```python
from build123d import *

# Parameters (mm, degrees)
EXTRUDE_1_DEPTH     = 5
SKETCH_2_W          = 5.436001784
SKETCH_2_H          = 4
CUT_EXTRUDE_1_DEPTH = 0.3
FILLET_2_R          = 0.3
EXTRUDE_2_DEPTH     = 5


with BuildPart() as part:
    # 草图1 → 凸台-拉伸1 (new body)
    with BuildSketch(Plane.XY):
        with BuildLine():
            Line((-6.127180226, -2.201181898), (-3.631722259, 2.12107809))
            ThreePointArc((-3.631722259, 2.12107809), (-3.262353303, 2.018731118), (-3.073540248, 1.685177587))
            Line((-3.073540248, 1.685177587), (1.998975947, -2.27609726))
            Line((1.998975947, -2.27609726), (6.288373272, -9.705551361))
            Line((6.288373272, -9.705551361), (7.418073814, -11.662250097))
            Line((7.418073814, -11.662250097), (2.221921391, -14.662250097))
            Line((2.221921391, -14.662250097), (-4.395129419, -3.201181898))
            Line((-4.395129419, -3.201181898), (-6.127180226, -2.201181898))
        make_face()
    extrude(amount=EXTRUDE_1_DEPTH)

    # 草图2 → 切除-拉伸1 (cut)
    with BuildSketch(Plane(origin=(-0.346861308, -0.444164989, 0), x_dir=(0.7881471083112889, -0.6154869094144516, 0), z_dir=(0.6154869094144517, 0.788147108311289, 0))):
        with Locations((-0.241605711, -2.5)):
            Rectangle(SKETCH_2_W, SKETCH_2_H)
    extrude(amount=-CUT_EXTRUDE_1_DEPTH, mode=Mode.SUBTRACT)

    # 圆角2
    fillet_2_edges = [part.edges().sort_by_distance(p)[0] for p in [
        (-2.864112767, 1.14099, 2.5),
        (-0.721928223, -0.531903969, 0.5),
        (1.42025632, -2.204797938, 2.5),
        (-0.721928223, -0.531903969, 4.5),
    ]]
    fillet(fillet_2_edges, radius=FILLET_2_R - 0.0001)  # a hair under: the kernel refuses the full size

    # 草图3 → 凸台-拉伸2 (add)
    with BuildSketch(Plane.XY.offset(5)):
        Polygon((7.418073814, -11.662250097), (15.362099483, -16.248735455), (13.872535789, -18.828735455), (4.438946425, -13.382250097), align=None)
    extrude(amount=-EXTRUDE_2_DEPTH)


solid = part.part
```
Build history of the part. All positions in model axes, mm. A direction names the side the tool comes from. Give positions to 0.01 mm unless a question says otherwise; leave off trailing zeros. Loops run counter-clockwise (first coordinate to the right, second up) from the corner with the lowest first, then second, coordinate; pieces in that order, holes last. Notation, with made-up numbers: (27.5, -39.75) -> (44.5, -39.75) arc R27 cw to (44.5, -12.75) -> close; hole circle Ø1 at (25.25, 76.5). An arc over 180 degrees is marked (long way). One line per question, with ' | ' between items.
Q1. Tool access for faces 1 (the flat face through (3.35, -14.01, 2.46)), 2 (the flat face through (-4.897, -0.07, 2.465)): list every direction of +Z, -Z, +X, -X, +Y, -Y with a clear straight run to the whole face (end or side of a thin tool).
Filled sheet:
face 1: +Z, -Z, -Y | face 2: +Z, -Z, -X, +Y
Q2. Drill centre lines: line 1 along X through (y, z) = (-14, 3); line 2 along X through (y, z) = (-6.5, 4.25); line 3 along Y through (x, z) = (-3.5, 3.6). Where is each one in solid material? Low to high. Write a range as [from, to].
Filled sheet:
line 1: x = [1.84, 3.37], [5.51, 11.47] | line 2: x = [-2.49, 4.44] | line 3: y = [-4.75, 2.12]
Q3. Pull direction Z, two halves, no side cores. Call faces 3 (the flat face through (-0.75, -0.51, 2.48)), 4 (the flat face through (3, -8, 5)), 5 (the flat face through (14.63, -17.52, 2.54)), 6 (the cylindrical face through (-0.636, -0.484, 0.586)): pulls with the +Z half, pulls with the -Z half, needs draft (parallel to the pull), parting line crosses it, or undercut.
Filled sheet:
face 3: undercut | face 4: pulls with the +Z half | face 5: needs draft | face 6: undercut
Q4. Cut at C-C, the plane y = -5.25. Write the cut outline in (x, z), plus the area to 3 significant figures.
Filled sheet:
outline: (-3.21, 0) -> (3.72, 0) -> (3.72, 5) -> (-3.21, 5) -> close | area: 34.6 mm²
Q5. Drop flat-ended pins along their axis: pin 1 (3 mm diameter, centred on y = -12.5, z = 2, fed in from -X); pin 2 (1 mm diameter, centred on y = -12, z = 3.5, fed in from +X); pin 3 (2 mm diameter, centred on y = -8.5, z = 2, fed in from -X); pin 4 (1 mm diameter, centred on x = -3, y = -10.5, fed in from -Z). Give the stop position or say it passes through.
Filled sheet:
pin 1: stops at x = 0.11 | pin 2: stops at x = 8.87 | pin 3: stops at x = -1.91 | pin 4: passes through
Q6. Cut at B-B, the plane x = 11. Write the cut outline in (y, z), plus the area to 3 significant figures.
Filled sheet:
outline: (-17.17, 0) -> (-13.73, 0) -> (-13.73, 5) -> (-17.17, 5) -> close | area: 17.2 mm²
